The model under review builds one solid part; all positions refer to its coordinate system, in mm. A direction names the side the tool comes from. Coordinates: 2 decimals unless noted, no trailing zeros. Order: outer loops, then holes, each group sorted by start corner. A loop starts at its lowest first (then second) coordinate and runs counter-clockwise, first axis right, second up. Notation, with made-up numbers: M 61.5,-1 L 99.5,-1 A30 ccw 99.5,36 Z; hole C 11.25,82 d6. An arc over 180 degrees is marked long. Answer as CSV lines item,"result". Start each with the question number.
Q1. Wall thickness on L1, parallel to Y at x = -6.25, z = 0.75; L2, parallel to X at y = 133, z = 0 (3 decimals); L3, parallel to Y at x = 5.75, z = 5.75: over which ranges is each line inside the solid? List them lowest first. Write a range as [from, to].
Q2. Consider section B-B on x = 0. Write out the cut boundary in (y, z) (3 decimals), and give its area (3 significant figures).
Q3. Consider section C-C on y = 50. Write out the cut boundary in (x, z), and give its area (3 significant figures).
Q4. For P1, Ø4, axis at x = -6.5, z = 3.5, coming from the +Y side; P2, Ø1.5, axis at x = -3.5, y = 158.5, coming from the +Z side; P3, Ø5, axis at x = 1, y = 105, coming from the -Z side (3 decimals); P4, Ø4, axis at y = 40, z = -8.5, coming from the -X side, all flat-tipped, find the tip position at first contact; note any pin that passes through.
Q5. Machinability: for faces 1 (the face through (-0.478, 220.212, -5.058)), 2 (the face through (4.141, 220.212, -2.943)), 3 (the face through (0.478, 220.212, 5.058)), 4 (the face through (5, 210.82, 2)), which of the approach directions +Z, -Z, +X, -X, +Y, -Y give a long, thin tool a straight path to every point of the face, cutting with its end or side? Answer none if there is none.
Q6. Consider section A-A on y = 125.5. Write out the cut boundary in (x, z) (3 decimals).
from build123d import *

# Parameters (mm, degrees)
SKETCH1_R           = 6.35
BOSS_EXTRUDE1_DEPTH = 421.64
SKETCH2_R           = 10.795
BOSS_EXTRUDE2_DEPTH = 421.64
SKETCH3_R           = 25.4
SKETCH3_R_2         = 6.35
CUT_EXTRUDE1_DEPTH  = 52.324
CUT_EXTRUDE2_START  = -57.658
SKETCH4_R           = 25.4
SKETCH4_R_2         = 6.35
CUT_EXTRUDE2_DEPTH  = 57.658
CHAMFER1_SIZE       = 6.35
SKETCH5_R           = 15.875
CUT_EXTRUDE4_DEPTH  = 212.372033273
BOSS_EXTRUDE3_DEPTH = 19.05


with BuildPart() as part:
    # Sketch1 → Boss-Extrude1 (new body)
    with BuildSketch(Plane(origin=(0, 0, 0), x_dir=(1, 0, 0), z_dir=(0, 1, 0))):
        with Locations(Location((0, 0, 0), (0, 0, 270))):
            Circle(SKETCH1_R)
    extrude(amount=BOSS_EXTRUDE1_DEPTH)

    # Sketch2 → Boss-Extrude2 (add)
    with BuildSketch(Plane(origin=(0, 0, 0), x_dir=(-1, 0, 0), z_dir=(0, -1, 0))):
        with Locations(Location((0, 0, 0), (0, 0, 90))):
            Circle(SKETCH2_R)
    extrude(amount=-BOSS_EXTRUDE2_DEPTH)

    # Sketch3 → Cut-Extrude1 (cut)
    with BuildSketch(Plane.XZ):
        Circle(SKETCH3_R)
        with Locations(Location((0, 0, 0), (0, 0, 270))):
            Circle(SKETCH3_R_2, mode=Mode.SUBTRACT)
    extrude(amount=-CUT_EXTRUDE1_DEPTH, mode=Mode.SUBTRACT)

    # Sketch4 → Cut-Extrude2 (cut)
    with BuildSketch(Plane(origin=(0, 421.64, 0), x_dir=(1, 0, 0), z_dir=(0, 1, 0)).offset(CUT_EXTRUDE2_START)):
        Circle(SKETCH4_R)
        with Locations(Location((0, 0, 0), (0, 0, 90))):
            Circle(SKETCH4_R_2, mode=Mode.SUBTRACT)
    extrude(amount=CUT_EXTRUDE2_DEPTH, mode=Mode.SUBTRACT)

    # Chamfer1
    # the kernel refuses this chamfer: 6.35 mm, written as the material it takes off along each edge
    with BuildSketch(Plane(origin=(0, 52.324, 0), x_dir=(0, 0, -1), z_dir=(-1, 0, 0))) as chamfer1_piece_1_section:
        Polygon((10.795, -CHAMFER1_SIZE), (10.795 - CHAMFER1_SIZE, 0), (10.795, 0), align=None)
    chamfer1_piece_1 = revolve(axis=Axis((0, 52.324, 0), (0, -1, 0)), mode=Mode.PRIVATE)
    chamfer1_piece_1 = chamfer1_piece_1 - Plane(origin=(0, 56.4676015, 0), x_dir=(0, 0, -1), z_dir=(0, -1, 0)) * Cylinder(6.35, 44, mode=Mode.PRIVATE)
    add(chamfer1_piece_1, mode=Mode.SUBTRACT)
    with BuildSketch(Plane(origin=(0, 363.982, 0), x_dir=(0, 0, -1), z_dir=(-1, 0, 0))) as chamfer1_piece_2_section:
        Polygon((10.795, CHAMFER1_SIZE), (10.795 - CHAMFER1_SIZE, 0), (10.795, 0), align=None)
    chamfer1_piece_2 = revolve(axis=Axis((0, 363.982, 0), (0, -1, 0)), mode=Mode.PRIVATE)
    chamfer1_piece_2 = chamfer1_piece_2 - Plane(origin=(0, 359.8383985, 0), x_dir=(0, 0, -1), z_dir=(0, -1, 0)) * Cylinder(6.35, 44, mode=Mode.PRIVATE)
    add(chamfer1_piece_2, mode=Mode.SUBTRACT)

    # Sketch5 → Cut-Extrude4 (cut, through all)
    with BuildSketch(Plane(origin=(0, 210.82, 0), x_dir=(1, 0, 0), z_dir=(0, 1, 0))):
        Circle(SKETCH5_R)
    extrude(amount=CUT_EXTRUDE4_DEPTH, mode=Mode.SUBTRACT)

    # Sketch6 → Boss-Extrude3 (add)
    with BuildSketch(Plane(origin=(0, 210.82, 0), x_dir=(1, 0, 0), z_dir=(0, 1, 0))):
        Polygon((-3.436763353, 4.753650281), (-5.83516358, -0.59949923), (-2.398400227, -5.353149511), (3.436763353, -4.753650281), (5.83516358, 0.59949923), (2.398400227, 5.353149511), align=None)
    extrude(amount=BOSS_EXTRUDE3_DEPTH)


solid = part.part
Evaluation:
1,L1,"y = [0, 210.82]"
1,L2,"x = [-10.795, 10.795]"
1,L3,"y = [56.01, 210.82]"
2,outline,"M 0,-6.35 L 54.229,-6.35 L 58.674,-10.795 L 210.82,-10.795 L 210.82,-5.107 L 229.87,-5.107 L 229.87,5.107 L 210.82,5.107 L 210.82,10.795 L 58.674,10.795 L 54.229,6.35 L 0,6.35 Z"
2,area,"4,240 mm²"
3,outline,"C 0,0 d12.7"
3,area,"127 mm²"
4,P1,"stops at y = 210.82"
4,P2,"stops at z = 10.44"
4,P3,"stops at z = -10.795"
4,P4,"passes through"
5,face 1,"-Z, -X, +Y"
5,face 2,"-Z, +X, +Y"
5,face 3,"+Z, +X, +Y"
5,face 4,"+Y"
6,outline,"C 0,0 d21.59"
